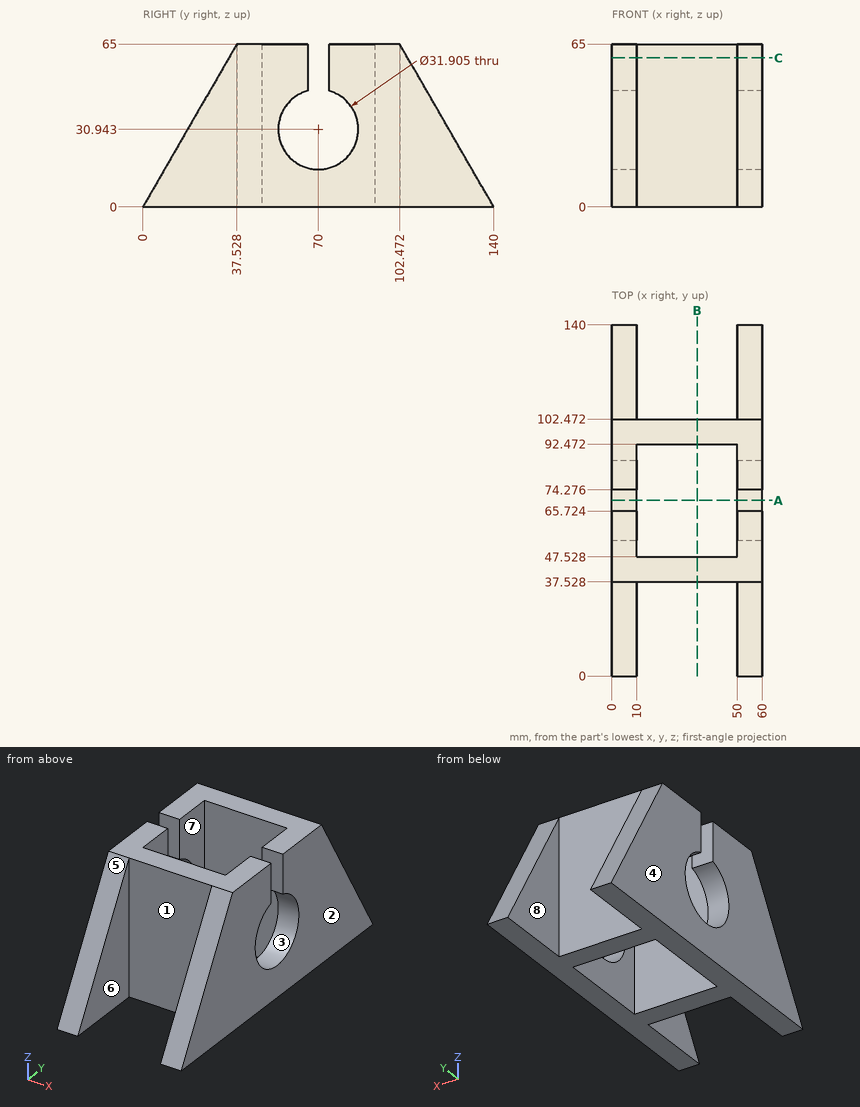
The figure shows three views and two pictorial views of one solid part (mm, origin at its lowest corner). Answer the questions. A direction names the side the tool comes from. Coordinates: 2 decimals unless noted, no trailing zeros. Write each loop counter-clockwise with the first axis right and the second up, starting at its lowest first coordinate (ties: lowest second). Pieces come first, ordered by that corner, then holes. Notation, with made-up numbers: (-22.75, -28) -> (26.25, -28) arc R26 ccw to (26.25, 9) -> close; hole circle Ø5 at (-28.75, 59). An arc over 180 degrees is marked (long way). Return JSON: item names as keys, results as strings.
(1) Which of the six approach directions +Z, -Z, +X, -X, +Y, -Y give full straight-line access (tool end or side, diameter ignored) to the marked faces 5, 6, 7 and 8?
Answers below:
{"face 5": "+Z, +X, -X, -Y", "face 6": "+Z, -Z, -Y", "face 7": "+Z, -Z", "face 8": "+Z, -Z, +Y"}
(2) Consider line 1 along Y through (x, z) = (24.5, 19); line 2 along X through (y, z) = (51, 30.5); line 3 along Y through (x, z) = (57, 54) (1 decimal). Determine where each line is inside the solid, lowest interval first. Write a range as from..to.
Answers below:
{"line 1": "37.53..47.53, 92.47..102.47", "line 2": "0..10, 50..60", "line 3": "31.2..65.7, 74.3..108.8"}
(3) The part is cut by section B-B on x = 34. Give the vertices of the cut face in (y, z), then the cut area to 3 significant figures.
Answers below:
{"outline": "(37.53, 0) -> (47.53, 0) -> (47.53, 65) -> (37.53, 65) -> close; (92.47, 0) -> (102.47, 0) -> (102.47, 65) -> (92.47, 65) -> close", "area": "1,300 mm^2"}
(4) Each of these flat-tipped pins is pushed along its axis until it touches: P1, Ø5, axis at x = 56.5, z = 53, coming from the -Y side; P2, Ø6, axis at x = 32, z = 10, coming from the +Y side; P3, Ø3, axis at x = 3, z = 53.5, coming from the -Y side. Where does it stop, or does it pass through?
Answers below:
{"P1": "y = 29.16", "P2": "y = 102.47", "P3": "y = 30.02"}
(5) The part is cut by section C-C on z = 59.5. Give the vertices of the cut face in (x, y), then the cut area to 4 significant figures.
Answers below:
{"outline": "(0, 34.35) -> (10, 34.35) -> (10, 37.53) -> (50, 37.53) -> (50, 34.35) -> (60, 34.35) -> (60, 65.72) -> (50, 65.72) -> (50, 47.53) -> (10, 47.53) -> (10, 65.72) -> (0, 65.72) -> close; (0, 74.28) -> (10, 74.28) -> (10, 92.47) -> (50, 92.47) -> (50, 74.28) -> (60, 74.28) -> (60, 105.65) -> (50, 105.65) -> (50, 102.47) -> (10, 102.47) -> (10, 105.65) -> (0, 105.65) -> close", "area": "2,055 mm^2"}
(6) The part is cut by section A-A on y = 70. Give the vertices of the cut face in (x, z), then the cut area to 3 significant figures.
Answers below:
{"outline": "(0, 0) -> (10, 0) -> (10, 14.99) -> (0, 14.99) -> close; (50, 0) -> (60, 0) -> (60, 14.99) -> (50, 14.99) -> close", "area": "300 mm^2"}
(7) For a pull along X with two mould halves and no side action, classify the marked faces 1, 2, 3 and 4 as pulls with the +X half, pulls with the -X half, needs draft (parallel to the pull), parting line crosses it, or undercut.
Answers below:
{"face 1": "undercut", "face 2": "pulls with the +X half", "face 3": "needs draft", "face 4": "pulls with the -X half"}
